from build123d import *

# Parameters (mm, degrees)
CROQUIS1_R              = 3.5
CROQUIS1_R_2            = 1.2
SALIENTE_EXTRUIR1_DEPTH = 1.25


with BuildPart() as part:
    # Croquis1 → Saliente-Extruir1 (new body, symmetric)
    with BuildSketch(Plane.XY):
        Polygon((-15, 18.5), (-8, 18.5), (-8, 16), (8, 16), (8, 18.5), (15, 18.5), (15, -18.5), (8, -18.5), (8, -16), (-8, -16), (-8, -18.5), (-15, -18.5), align=None)
        Circle(CROQUIS1_R, mode=Mode.SUBTRACT)
        with Locations((0, 7.5)):
            Circle(CROQUIS1_R_2, mode=Mode.SUBTRACT)
        with Locations((5.303300859, 5.303300859)):
            Circle(CROQUIS1_R_2, mode=Mode.SUBTRACT)
        with Locations((7.5, 0)):
            Circle(CROQUIS1_R_2, mode=Mode.SUBTRACT)
        with Locations((5.303300859, -5.303300859)):
            Circle(CROQUIS1_R_2, mode=Mode.SUBTRACT)
        with Locations((0, -7.5)):
            Circle(CROQUIS1_R_2, mode=Mode.SUBTRACT)
        with Locations((-5.303300859, -5.303300859)):
            Circle(CROQUIS1_R_2, mode=Mode.SUBTRACT)
        with Locations((-7.5, 0)):
            Circle(CROQUIS1_R_2, mode=Mode.SUBTRACT)
        with Locations((-5.303300859, 5.303300859)):
            Circle(CROQUIS1_R_2, mode=Mode.SUBTRACT)
    extrude(amount=SALIENTE_EXTRUIR1_DEPTH, both=True)


solid = part.part
Model file for the job. Use its own axes, mm. A direction names the side the tool comes from. Round coordinates to 2 decimals unless told otherwise and drop trailing zeros. Loops run counter-clockwise (first coordinate to the right, second up) from the corner with the lowest first, then second, coordinate; pieces in that order, holes last.
1. Band-saw the part on D-D, the plane x = 0. List the corners of the cut face in (y, z), and give its area (3 significant figures).
Check values:
outline: (-16, -1.25) - (-8.7, -1.25) - (-8.7, 1.25) - (-16, 1.25) - close; (-6.3, -1.25) - (-3.5, -1.25) - (-3.5, 1.25) - (-6.3, 1.25) - close; (3.5, -1.25) - (6.3, -1.25) - (6.3, 1.25) - (3.5, 1.25) - close; (8.7, -1.25) - (16, -1.25) - (16, 1.25) - (8.7, 1.25) - close
area: 50.5 mm2
2. Mould opens along X. For faces 4 (the flat face through (0, -16, 0)), 5 (the flat face through (-12, 18.5, 0)), 6 (the flat face through (15, 0, 0)) say: +X half, -X half, draft (parallel to the pull), parting line (faces both ways), or undercut.
Check values:
face 4: undercut
face 5: draft
face 6: +X half
3. Band-saw the part on B-B, the plane x = -7.5. List the corners of the cut face in (y, z).
Check values:
outline: (-16, -1.25) - (-1.2, -1.25) - (-1.2, 1.25) - (-16, 1.25) - close; (1.2, -1.25) - (16, -1.25) - (16, 1.25) - (1.2, 1.25) - close
4. Band-saw the part on A-A, the plane y = 0. List the corners of the cut face in (x, z).
Check values:
outline: (-15, -1.25) - (-8.7, -1.25) - (-8.7, 1.25) - (-15, 1.25) - close; (-6.3, -1.25) - (-3.5, -1.25) - (-3.5, 1.25) - (-6.3, 1.25) - close; (3.5, -1.25) - (6.3, -1.25) - (6.3, 1.25) - (3.5, 1.25) - close; (8.7, -1.25) - (15, -1.25) - (15, 1.25) - (8.7, 1.25) - close
5. Drop a flat-ended pin along its axis: P1, Ø1, axis at x = 0.5, z = 0.5, coming from the +Y side. Give the stop position or say it passes through.
Check values:
P1: stops at y = 16
6. Tool access for faces 1 (the cylindrical face through (4.35, -6.03, -0.02)), 2 (the flat face through (-8, -17, 0)), 3 (the flat face through (8, 17, 0)): list every direction of +Z, -Z, +X, -X, +Y, -Y with a clear straight run to the whole face (end or side of a thin tool).
Check values:
face 1: +Z, -Z
face 2: +Z, -Z, -Y
face 3: +Z, -Z, +Y
7. Wall check: probe 1 along Y at (x, z) = (0, 0.1); probe 2 along Y at (x, z) = (7.5, 0.7); probe 3 along Y at (x, z) = (0.75, 0.7). Give the ranges that are in metal, low to high.
Check values:
probe 1: y = -16 to -8.7, -6.3 to -3.5, 3.5 to 6.3, 8.7 to 16
probe 2: y = -16 to -1.2, 1.2 to 16
probe 3: y = -16 to -8.44, -6.56 to -3.42, 3.42 to 6.56, 8.44 to 16
8. Band-saw the part on C-C, the plane y = -7.5. List the corners of the cut face in (x, z), and give its area (3 significant figures).
Check values:
outline: (-15, -1.25) - (-1.2, -1.25) - (-1.2, 1.25) - (-15, 1.25) - close; (1.2, -1.25) - (15, -1.25) - (15, 1.25) - (1.2, 1.25) - close
area: 69.0 mm2
